Input: part model. Units: mm. Frame: model coordinates. A direction names the side the tool comes from. Give positions to 0.01 mm unless a question says otherwise; leave off trailing zeros. Order: outer loops, then holes, each group sorted by start corner. A loop starts at its lowest first (then second) coordinate and runs counter-clockwise, first axis right, second up.
```python
from build123d import *

# Parameters (mm, degrees)
BOSS_EXTRUDE1_DEPTH    = 23
BOSS_EXTRUDE2_DEPTH    = 11
BOSS_EXTRUDE3_START    = 5
SKETCH1_4_R            = 5
BOSS_EXTRUDE3_DEPTH    = 6
BOSS_EXTRUDE4_START    = -12
SKETCH1_5_R            = 5
BOSS_EXTRUDE4_DEPTH    = 6
BOSS_EXTRUDE5_DEPTH    = 9
FILLET1_RADIUS         = 9
FILLET1_LENGTH         = 6
FILLET2_RADIUS         = 9
FILLET2_LENGTH         = 6
F_10_0MM_DOWEL_HOLE1_D = 10


with BuildPart() as part:
    # Sketch1 → Boss-Extrude1 (new, symmetric)
    with BuildSketch(Plane.XY):
        with BuildLine():
            ThreePointArc((6, 16.970562748), (-6.763446053, 16.681001094), (-16.124515497, 8))
            ThreePointArc((-16.124515497, 8), (-17.269106839, 5.077198931), (-17.88854382, 2))
            Line((-17.88854382, 2), (-12.845232579, 2))
            ThreePointArc((-12.845232579, 2), (13, 0), (-12.845232579, -2))
            Line((-12.845232579, -2), (-17.88854382, -2))
            ThreePointArc((-17.88854382, -2), (-17.269106839, -5.077198931), (-16.124515497, -8))
            ThreePointArc((-16.124515497, -8), (-6.763446053, -16.681001094), (6, -16.970562748))
            ThreePointArc((6, -16.970562748), (18, 0), (6, 16.970562748))
        make_face()
    extrude(amount=BOSS_EXTRUDE1_DEPTH, both=True)

    # Sketch1<3> → Boss-Extrude2 (add, symmetric)
    with BuildSketch(Plane.XY):
        with BuildLine():
            Line((21, 11.66726189), (6, 16.970562748))
            ThreePointArc((6, 16.970562748), (18, 0), (6, -16.970562748))
            Line((6, -16.970562748), (21, -11.66726189))
            Line((21, -11.66726189), (21, 11.66726189))
        make_face()
    extrude(amount=BOSS_EXTRUDE2_DEPTH, both=True)

    # Sketch1<4> → Boss-Extrude3 (add)
    with BuildSketch(Plane.XY.offset(BOSS_EXTRUDE3_START)):
        with BuildLine():
            Line((35.333333333, 6.599663291), (21, 11.66726189))
            Line((21, 11.66726189), (21, -11.66726189))
            Line((21, -11.66726189), (35.333333333, -6.599663291))
            ThreePointArc((35.333333333, -6.599663291), (40, 0), (35.333333333, 6.599663291))
        make_face()
        with Locations((33, 0)):
            Circle(SKETCH1_4_R, mode=Mode.SUBTRACT)
    extrude(amount=BOSS_EXTRUDE3_DEPTH)

    # Sketch1<5> → Boss-Extrude4 (add)
    with BuildSketch(Plane.XY.offset(BOSS_EXTRUDE4_START)):
        with BuildLine():
            Line((35.333333333, 6.599663291), (21, 11.66726189))
            Line((21, 11.66726189), (21, -11.66726189))
            Line((21, -11.66726189), (35.333333333, -6.599663291))
            ThreePointArc((35.333333333, -6.599663291), (40, 0), (35.333333333, 6.599663291))
        make_face()
        with Locations((33, 0)):
            Circle(SKETCH1_5_R, mode=Mode.SUBTRACT)
    extrude(amount=BOSS_EXTRUDE4_DEPTH)

    # Sketch1<6> → Boss-Extrude5 (add, symmetric)
    with BuildSketch(Plane.XY):
        with BuildLine():
            ThreePointArc((-17.88854382, 2), (-17.269106839, 5.077198931), (-16.124515497, 8))
            Line((-16.124515497, 8), (-33, 8))
            Line((-33, 8), (-33, 2))
            Line((-33, 2), (-17.88854382, 2))
        make_face()
        with BuildLine():
            Line((-33, -8), (-16.124515497, -8))
            ThreePointArc((-16.124515497, -8), (-17.269106839, -5.077198931), (-17.88854382, -2))
            Line((-17.88854382, -2), (-33, -2))
            Line((-33, -2), (-33, -8))
        make_face()
    extrude(amount=BOSS_EXTRUDE5_DEPTH, both=True)

    # Fillet1: full round fillet: the end face becomes a half cylinder, R = half its width
    fillet1_face = Plane((-33, 5, 0), x_dir=(0, -1, 0), z_dir=(-1, 0, 0))  # on the end face: x along it, z out of the body
    fillet1_slab = fillet1_face.offset(-FILLET1_RADIUS / 2) * Box(FILLET1_LENGTH, 2 * FILLET1_RADIUS, FILLET1_RADIUS, mode=Mode.PRIVATE)  # the body's end, R deep
    fillet1_round = Plane((-24, 5, 0), x_dir=(-1, 0, 0), z_dir=(0, -1, 0)) * Cylinder(FILLET1_RADIUS, FILLET1_LENGTH, mode=Mode.PRIVATE)  # its axis R under the face
    add(fillet1_slab - fillet1_round, mode=Mode.SUBTRACT)

    # Fillet2: full round fillet: the end face becomes a half cylinder, R = half its width
    fillet2_face = Plane((-33, -5, 0), x_dir=(0, 1, 0), z_dir=(-1, 0, 0))  # on the end face: x along it, z out of the body
    fillet2_slab = fillet2_face.offset(-FILLET2_RADIUS / 2) * Box(FILLET2_LENGTH, 2 * FILLET2_RADIUS, FILLET2_RADIUS, mode=Mode.PRIVATE)  # the body's end, R deep
    fillet2_round = Plane((-24, -5, 0), x_dir=(-1, 0, 0), z_dir=(0, 1, 0)) * Cylinder(FILLET2_RADIUS, FILLET2_LENGTH, mode=Mode.PRIVATE)  # its axis R under the face
    add(fillet2_slab - fillet2_round, mode=Mode.SUBTRACT)

    # Ø10.0mm Dowel Hole1 (through all)
    with Locations(Plane(origin=(-24, 8, 0), x_dir=(1, 0, 0), z_dir=(0, 1, 0))):
        with Locations((0, 0)):
            Hole(F_10_0MM_DOWEL_HOLE1_D / 2)


solid = part.part
```
1) Line query: probe 1 along Y at (x, z) = (-29, -2); probe 2 along X at (y, z) = (5, -2); probe 3 along Z at (x, y) = (-24, -5.2). Output: solid intervals per line, ascending.
2) Cut plane D-D (x = -25.5). Return the cut outline in (y, z).
3) Cut plane C-C (z = 20). Return the cut outline in (x, y).
4) Pull-direction query (Y, two-part tool) for faces 4 (the face through (-18, -2, 0)), 5 (the face through (40, 0, 8)), 6 (the face through (-19, -5, 0)), 7 (the face through (-18.8, 8, -0.1)); classes: pulls with the +Y half, pulls with the -Y half, needs draft (parallel to the pull), parting line crosses it, or undercut.
5) Reachability of faces 1 (the face through (26, 0, -12)), 2 (the face through (26, 0, 5)), 3 (the face through (-19, -8, 2)) from +Z, -Z, +X, -X, +Y, -Y: full face, straight path, thin tool, end or side. Return the list, or none.
6) First-contact query: P1, Ø1, axis at y = 5.5, z = -4, coming from the +X side; P2, Ø21, axis at x = 0, y = 0, coming from the +Z side; P3, Ø1.1, axis at y = 4, z = -11.5, coming from the -X side; P4, Ø1, axis at y = -5.5, z = 8, coming from the -X side. Flat tips, straight axial feed; report the tip coordinate or a pass-through.
7) Cut plane A-A (x = 0). Return the cut outline in (y, z).
8) Cut plane B-B (y = -3). Count the separate pieces of the cut face and the enclosed holes in it, then the cut area to 3 significant figures.
Geometry says:
1. probe 1: y = -8 to -2, 2 to 8
1. probe 2: x = -32.77 to -28.58, -19.42 to -12, 12 to 21
1. probe 3: z = -9 to -5, 5 to 9
2. outline: (-8, -8.87) - (-2, -8.87) - (-2, -4.77) - (-8, -4.77) - close; (-8, 4.77) - (-2, 4.77) - (-2, 8.87) - (-8, 8.87) - close; (2, -8.87) - (8, -8.87) - (8, -4.77) - (2, -4.77) - close; (2, 4.77) - (8, 4.77) - (8, 8.87) - (2, 8.87) - close
3. outline: (-17.89, -2) arc R18 ccw (long way) to (-17.89, 2) - (-12.85, 2) arc R13 cw (long way) to (-12.85, -2) - close
4. face 4: undercut
4. face 5: parting line crosses it
4. face 6: needs draft
4. face 7: pulls with the +Y half
5. face 1: -Z, +X, +Y, -Y
5. face 2: +X, +Y, -Y
5. face 3: +Z, -Z, -X, -Y
6. P1: stops at x = 21
6. P2: passes through
6. P3: stops at x = -17.67
6. P4: stops at x = -28.97
7. outline: (-18, -23) - (-13, -23) - (-13, 23) - (-18, 23) - close; (13, -23) - (18, -23) - (18, 23) - (13, 23) - close
8. separate pieces: 4
8. enclosed holes: 1
8. area: 826 mm2
